Geometry check sheet. Reference: drawing and pictorial views, mm from the part's lowest x, y, z. Coordinates: 2 decimals unless noted, no trailing zeros. Order: outer loops, then holes, each group sorted by start corner. A loop starts at its lowest first (then second) coordinate and runs counter-clockwise, first axis right, second up. Notation, with made-up numbers: M -30.5,26 L -0.5,26 A23 cw -0.5,40 Z; hole C 13,20.5 d4. An arc over 180 degrees is marked long. Return JSON: item names as keys, results as strings.
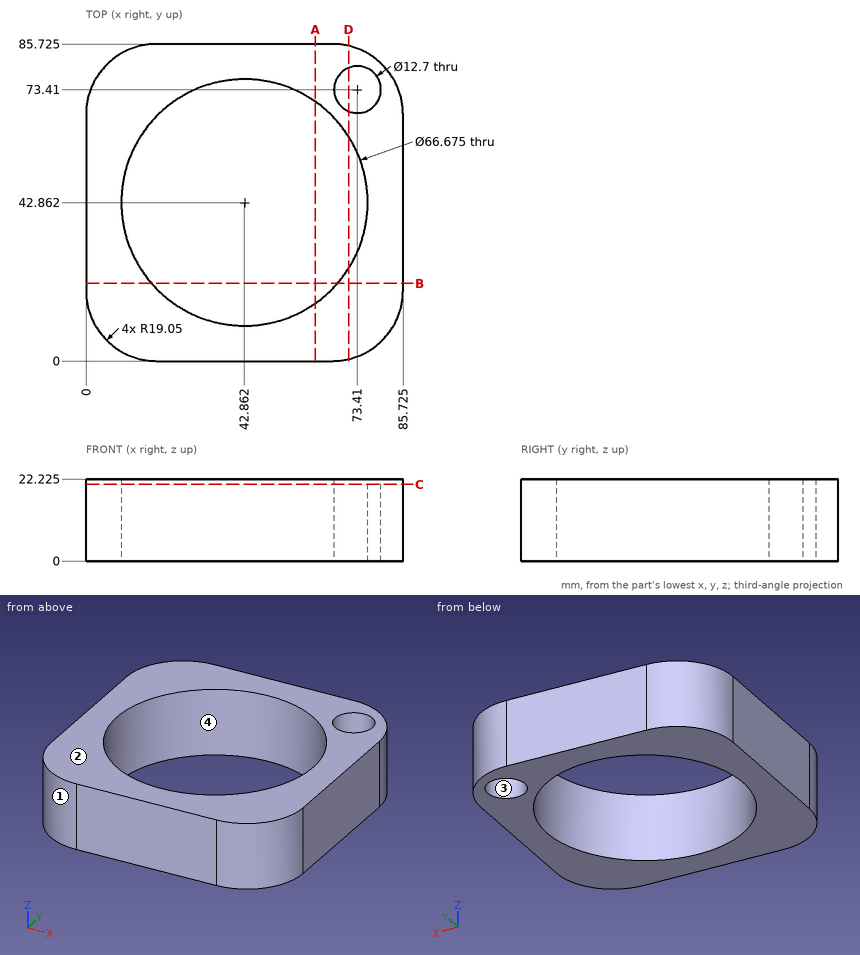
Q1. Cross-section at D-D, the plane x = 71. Record the boundary of the cut face in (y, z) (1 decimal).
Values:
{"outline": "M 0.5,0 L 25,0 L 25,22.2 L 0.5,22.2 Z; M 60.7,0 L 67.5,0 L 67.5,22.2 L 60.7,22.2 Z; M 79.3,0 L 85.2,0 L 85.2,22.2 L 79.3,22.2 Z"}
Q2. Go/stop test with flat-tipped pins: pin 1 (10 mm diameter, centred on x = 17.5, y = 59, fed in from +Z) (1 decimal); pin 2 (3 mm diameter, centred on x = 16.5, z = 6, fed in from +Y); pin 3 (3 mm diameter, centred on y = 14, z = 17.5, fed in from -X). Record where each tip stops, or that it passes through.
Values:
{"pin 1": "z = 22.2", "pin 2": "y = 85.7", "pin 3": "x = 0.33"}
Q3. Cross-section at A-A, the plane x = 62. Record the boundary of the cut face in (y, z) (1 decimal), and give its area (3 significant figures).
Values:
{"outline": "M 0,0 L 15.6,0 L 15.6,22.2 L 0,22.2 Z; M 70.2,0 L 85.7,0 L 85.7,22.2 L 70.2,22.2 Z", "area": "692 mm^2"}
Q4. Draft check along Y on the marked faces 1, 2, 3 and 4. Enter one of: pulls with the +Y half, pulls with the -Y half, needs draft (parallel to the pull), parting line crosses it, or undercut.
Values:
{"face 1": "pulls with the -Y half", "face 2": "needs draft", "face 3": "undercut", "face 4": "undercut"}
Q5. Cross-section at C-C, the plane z = 20.75. State how many separate pieces and enclosed holes the cut face has, and give its area (3 significant figures).
Values:
{"separate pieces": "1", "enclosed holes": "2", "area": "3,420 mm^2"}
Q6. Material ranges on line 1 along X through (y, z) = (72.5, 19.25) (1 decimal); line 2 along X through (y, z) = (69, 11.5) (1 decimal); line 3 along Y through (x, z) = (55.5, 13.25) (1 decimal), recorded low to high.
Values:
{"line 1": "0.9 to 27.6, 58.1 to 67.1, 79.7 to 84.8", "line 2": "0.1 to 22.2, 63.6 to 68.8, 78 to 85.6", "line 3": "0 to 12, 73.7 to 85.7"}
Q7. Cross-section at B-B, the plane y = 21. Record the boundary of the cut face in (x, z) (1 decimal).
Values:
{"outline": "M 0,0 L 17.7,0 L 17.7,22.2 L 0,22.2 Z; M 68,0 L 85.7,0 L 85.7,22.2 L 68,22.2 Z"}
